Read the model definition and answer for the solid it produces. Units are mm, in the model's axes. Face numbers are marked on the shaded views. A direction names the side the tool comes from. Coordinates: 2 decimals unless noted, no trailing zeros. Order: outer loops, then holes, each group sorted by start corner. A loop starts at its lowest first (then second) coordinate and runs counter-clockwise, first axis right, second up. Notation, with made-up numbers: (-33.75, -18.5) -> (1.25, -18.5) arc R22 ccw to (1.25, 13.5) -> close; hole circle Ø1 at (75, 5). An arc over 180 degrees is marked (long way). Answer as a JSON object with one key per item and string values. Group by question number.
1) Section B-B on x = 9.5 is taken. Count the separate pieces of the cut face and the enclosed holes in it, and give its area (3 significant figures).
2) Section C-C on z = 17.5 is taken. Determine the outline of the cut face in (x, y), and give its area (3 significant figures).
3) Section D-D on x = 2.4 is taken. Determine the outline of the cut face in (y, z), and give its area (3 significant figures).
4) Given pin 1 (2.5 mm diameter, centred on y = -25.45, z = 14.95, fed in from -X); pin 2 (5 mm diameter, centred on y = -20.5, z = 10, fed in from -X), each flat-ended and moving along its own axis, determine where each tip first touches the part or whether it passes through.
5) A tool of negligible diameter and unlimited length cuts with its end or side. For the marked faces 4 and 5, from which of +Z, -Z, +X, -X, +Y, -Y can it reach the whole face along a straight path? Write none if from no direction.
6) Determine the mould class of the marked faces 1, 2 and 3 for opening direction Y: released by +Y, released by -Y, zero draft, split by the parting line, or undercut.
7) Section A-A on y = -20.5 is taken. Determine the outline of the cut face in (x, z).
8) Consider L1, parallel to Y at x = 13, z = 5.5; L2, parallel to Z at x = 16.65, y = -20.5; L3, parallel to X at y = -39.5, z = 7.25. Determine where each line is inside the solid, lowest interval first.
from build123d import *

# Parameters (mm, degrees)
SKETCH_1_W          = 12
SKETCH_1_H          = 20
SKETCH_1_R          = 1.2
EXTRUDE_1_DEPTH     = 1.5
EXTRUDE_2_DEPTH     = 20
SKETCH_3_R          = 1.5
CUT_EXTRUDE_1_DEPTH = 10
FILLET_1_R          = 2
FILLET_2_R          = 1


with BuildPart() as part:
    # 草图1 → 凸台-拉伸1 (new body)
    with BuildSketch(Plane(origin=(0, 0, 0), x_dir=(1, 0, 0), z_dir=(0, 1, 0))):
        with Locations((6, -10)):
            Rectangle(SKETCH_1_W, SKETCH_1_H)
        with Locations(Location((2.4, -3, 0), (0, 0, 270))):
            Circle(SKETCH_1_R, mode=Mode.SUBTRACT)
        with Locations(Location((9.5, -2.5, 0), (0, 0, 270))):
            Circle(SKETCH_1_R, mode=Mode.SUBTRACT)
        with Locations(Location((2.4, -17, 0), (0, 0, 270))):
            Circle(SKETCH_1_R, mode=Mode.SUBTRACT)
        with Locations(Location((9.5, -10, 0), (0, 0, 270))):
            Circle(SKETCH_1_R, mode=Mode.SUBTRACT)
        with Locations(Location((9.5, -17.5, 0), (0, 0, 270))):
            Circle(SKETCH_1_R, mode=Mode.SUBTRACT)
    extrude(amount=EXTRUDE_1_DEPTH)

    # 草图2 → 凸台-拉伸2 (add)
    with BuildSketch(Plane(origin=(0, 0, 0), x_dir=(-1, 0, 0), z_dir=(0, 0, -1))):
        Polygon((-16, -20.5), (-16, 0), (-12, 0), (-12, 1.5), (-17.5, 1.5), (-17.5, -20.5), align=None)
    extrude(amount=-EXTRUDE_2_DEPTH)

    # 镜向2: part across plane


with BuildPart() as part_1:
    add(part.part)
    add(part.part.mirror(Plane(origin=(0, -20.5, 20), x_dir=(0, 0, 1), z_dir=(0, -1, 0))))

    # 草图3 → 切除-拉伸1 (cut)
    with BuildSketch(Plane(origin=(17.5, 0, 0), x_dir=(0, 0, -1), z_dir=(1, 0, 0))):
        with Locations(Location((-10, -20.5, 0), (0, 0, 90))):
            Circle(SKETCH_3_R)
        with Locations(Location((-14.949747468, -15.550252532, 0), (0, 0, 90))):
            Circle(SKETCH_3_R)
        with Locations(Location((-5.050252532, -15.550252532, 0), (0, 0, 90))):
            Circle(SKETCH_3_R)
        with Locations(Location((-5.050252532, -25.449747468, 0), (0, 0, 90))):
            Circle(SKETCH_3_R)
        with Locations(Location((-14.949747468, -25.449747468, 0), (0, 0, 90))):
            Circle(SKETCH_3_R)
    extrude(amount=-CUT_EXTRUDE_1_DEPTH, mode=Mode.SUBTRACT)

    # 圆角1
    fillet_1_edges = [part_1.edges().sort_by_distance(p)[0] for p in [
        (17.5, 1.5, 10),
        (17.5, -42.5, 10),
    ]]
    fillet(fillet_1_edges, radius=FILLET_1_R)

    # 圆角2
    fillet_2_edges = [part_1.edges().sort_by_distance(p)[0] for p in [
        (16, 0, 10),
        (16, -41, 10),
    ]]
    fillet(fillet_2_edges, radius=FILLET_2_R)


solid = part_1.part
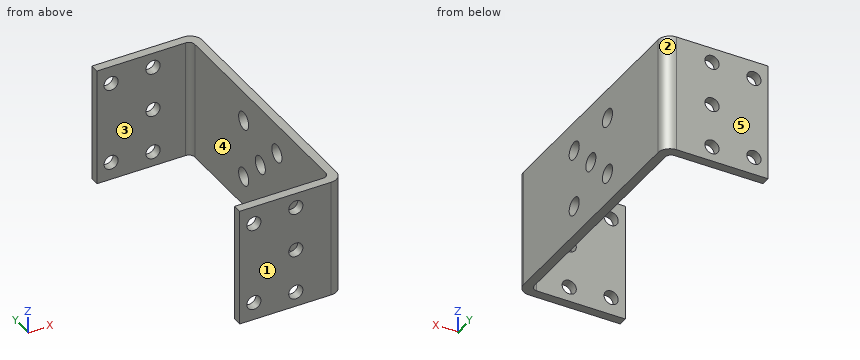
Worked answers:
{
 "1": {"separate pieces": "8", "enclosed holes": "0", "area": "38.4 mm²"},
 "2": {"outline": "(0, -42.5) -> (1.31, -42.5) -> (1.31, -41) -> (0, -41) -> close; (0, 0) -> (1.31, 0) -> (1.31, 1.5) -> (0, 1.5) -> close; (3.49, -42.5) -> (8.3, -42.5) -> (8.3, -41) -> (3.49, -41) -> close; (3.49, 0) -> (8.3, 0) -> (8.3, 1.5) -> (3.49, 1.5) -> close; (10.7, -42.5) -> (15.5, -42.5) arc R2 ccw to (17.5, -40.5) -> (17.5, -0.5) arc R2 ccw to (15.5, 1.5) -> (10.7, 1.5) -> (10.7, 0) -> (15, 0) arc R1 cw to (16, -1) -> (16, -40) arc R1 cw to (15, -41) -> (10.7, -41) -> close", "area": "99.0 mm²"},
 "3": {"outline": "(-42.5, 0) -> (-41, 0) -> (-41, 1.8) -> (-42.5, 1.8) -> close; (-42.5, 4.2) -> (-41, 4.2) -> (-41, 15.8) -> (-42.5, 15.8) -> close; (-42.5, 18.2) -> (-41, 18.2) -> (-41, 20) -> (-42.5, 20) -> close; (0, 0) -> (1.5, 0) -> (1.5, 1.8) -> (0, 1.8) -> close; (0, 4.2) -> (1.5, 4.2) -> (1.5, 15.8) -> (0, 15.8) -> close; (0, 18.2) -> (1.5, 18.2) -> (1.5, 20) -> (0, 20) -> close", "area": "45.6 mm²"},
 "4": {"pin 1": "passes through", "pin 2": "stops at x = 16"},
 "5": {"face 4": "+Z, -Z, -X", "face 5": "+Z, -Z, +X, -X, +Y"},
 "6": {"face 1": "released by -Y", "face 2": "released by +Y", "face 3": "undercut"},
 "7": {"outline": "(16, 0) -> (17.5, 0) -> (17.5, 8.5) -> (16, 8.5) -> close; (16, 11.5) -> (17.5, 11.5) -> (17.5, 20) -> (16, 20) -> close"},
 "8": {"L1": "y = -42.5 to -41, 0 to 1.5", "L2": "z = 0 to 8.5, 11.5 to 20", "L3": "x = 16 to 17.5"}
}
